```python
from build123d import *

# Parameters (mm, degrees)
SKETCH1_W               = 15
SKETCH1_H               = 32
SKETCH1_R               = 0.55
SKETCH1_W_2             = 12.4
SKETCH1_H_2             = 22.8
SERVO_MOUNT_PLATE_DEPTH = 4
SKETCH3_R               = 0.55
BOSS_EXTRUDE3_DEPTH     = 25
BOSS_EXTRUDE9_DEPTH     = 15
CUT_EXTRUDE3_START      = 1.5
CUT_EXTRUDE3_DEPTH      = 13.5
FILLET1_R               = 3
BODY_MOVE_COPY1_ANGLE   = 90


with BuildPart() as part:
    # Sketch1 → Servo Mount Plate (new body)
    with BuildSketch(Plane.XY):
        Rectangle(SKETCH1_W, SKETCH1_H)
        with Locations((0, 13.9)):
            Circle(SKETCH1_R, mode=Mode.SUBTRACT)
        with Locations((0, -13.9)):
            Circle(SKETCH1_R, mode=Mode.SUBTRACT)
        Rectangle(SKETCH1_W_2, SKETCH1_H_2, mode=Mode.SUBTRACT)
    extrude(amount=SERVO_MOUNT_PLATE_DEPTH)

    # Sketch3 → Boss-Extrude3 (add)
    # profile 1 of 2: a face of its own
    with BuildSketch(Plane.XY.offset(4)):
        Polygon((6.2, -11.4), (-6.2, -11.4), (-7.5, -11.4), (-7.5, -16), (7.5, -16), (7.5, -11.4), align=None)
        with Locations((0, -13.9)):
            Circle(SKETCH3_R, mode=Mode.SUBTRACT)
    # profile 2 of 2: a face of its own
    with BuildSketch(Plane.XY.offset(4)):
        with Locations((0, -13.9)):
            Circle(SKETCH3_R)
    extrude(amount=BOSS_EXTRUDE3_DEPTH)

    # Sketch5 → Boss-Extrude9 (add)
    with BuildSketch(Plane.XY.offset(14)):
        with BuildLine():
            Line((5.615385478, -4.685808185), (7.5, -6.00542948))
            Line((7.5, -6.00542948), (21.773725966, -16))
            Line((21.773725966, -16), (21.773725966, -5.013028701))
            Line((21.773725966, -5.013028701), (11.126345195, 2.442347577))
            ThreePointArc((11.126345195, 2.442347577), (9.098023831, -1.683915153), (5.615385478, -4.685808185))
        make_face()
        Polygon((21.773725966, -16), (7.5, -6.00542948), (7.5, -11.4), (7.5, -16), align=None)
        with BuildLine():
            Line((7.5, -11.4), (7.5, -6.00542948))
            Line((7.5, -6.00542948), (5.615385478, -4.685808185))
            ThreePointArc((5.615385478, -4.685808185), (0.865900109, -6.117354403), (-4.044697914, -5.415241232))
            Line((-4.044697914, -5.415241232), (-7.5, -11.4))
            Line((-7.5, -11.4), (7.5, -11.4))
        make_face()
    extrude(amount=BOSS_EXTRUDE9_DEPTH)

    # Sketch5<8> → Cut-Extrude3 (cut)
    with BuildSketch(Plane.XY.offset(14).offset(CUT_EXTRUDE3_START)):
        with BuildLine():
            Line((5.615385478, -4.685808185), (7.5, -6.00542948))
            Line((7.5, -6.00542948), (21.773725966, -16))
            Line((21.773725966, -16), (21.773725966, -5.013028701))
            Line((21.773725966, -5.013028701), (11.126345195, 2.442347577))
            ThreePointArc((11.126345195, 2.442347577), (9.098023831, -1.683915153), (5.615385478, -4.685808185))
        make_face()
    extrude(amount=CUT_EXTRUDE3_DEPTH, mode=Mode.SUBTRACT)

    # Fillet1
    fillet1_edges = [part.edges().sort_by_distance(p)[0] for p in [
        (6.85, -11.4, 4),
        (-6.85, -11.4, 4),
        (11.126345195, 2.442347577, 14.75),
        (21.773725966, -5.013028701, 14.75),
    ]]
    fillet(fillet1_edges, radius=FILLET1_R)


with BuildPart() as part_1:
    # Body-Move/Copy1: moved
    add(part.part.rotate(Axis((0, 0, 14.5), (1, 0, 0)), BODY_MOVE_COPY1_ANGLE))


solid = part_1.part
```
Verification items for the finished model (mm, model axes). A direction names the side the tool comes from. Give positions to 0.01 mm unless a question says otherwise; leave off trailing zeros. Order: outer loops, then holes, each group sorted by start corner. A loop starts at its lowest first (then second) coordinate and runs counter-clockwise, first axis right, second up. Notation, with made-up numbers: M 86.25,67.25 L 121.25,67.25 A15 ccw 121.25,94.25 Z; hole C 44,51.25 d8. An arc over 180 degrees is marked long. Return JSON: item names as keys, results as strings. Group by question number.
1) Section check A-A on z = 17. Record the cut outline in (x, y).
2) Mould release check, pull along X, two halves, no side actions. Record for faces 4 (the face through (-5.75, -6.9, 6.13)), 5 (the face through (0, 10.5, 0.6)), 6 (the face through (11.834, -0.261, 15.314)), 7 (the face through (6.84, 9.6, 3.96)): pulls with the +X half, pulls with the -X half, needs draft (parallel to the pull), parting line crosses it, or undercut.
3) Scan lines: line 1 (Z direction, x = 0, y = 13.1); line 2 (X direction, y = 12.5, z = 14.5); line 3 (X direction, y = 13.45, z = 28.4). Record each from-to range of solid material in increasing order.
4) Go/stop test with flat-tipped pins: pin 1 Ø4 at (x, y) = (15, -5.5) entering from +Z; pin 2 Ø12 at (x, y) = (6.5, -2) entering from +Z; pin 3 Ø7 at (y, z) = (10, 12.5) entering from +X. Record where each tip stops, or that it passes through.
5) Access from +Z, -Z, +X, -X, +Y, -Y to the whole of each face (thin tool, end or side, straight path). Record for faces 1 (the face through (-6.86, 9.6, 3.96)), 2 (the face through (15, -1, 9)), 3 (the face through (6.2, 13, 14)).
6) Section check B-B on x = -1.75. Record the cut outline in (y, z).
7) Section check D-D on y = 2.5. Record the cut outline in (x, z).
8) Section check C-C on z = 28.4. Record the cut outline in (x, y), and give its area (3 significant figures).
Answer block:
{
 "1": {"outline": "M -7.5,10.5 L -6.2,10.5 L -6.2,14.5 L -7.5,14.5 Z; M 6.2,10.5 L 7.5,10.5 L 7.5,14.5 L 6.2,14.5 Z"},
 "2": {"face 4": "pulls with the -X half", "face 5": "undercut", "face 6": "parting line crosses it", "face 7": "needs draft"},
 "3": {"line 1": "z = -1.5 to 0.05, 1.15 to 3.1, 25.9 to 27.85, 28.95 to 30.5", "line 2": "x = -7.5 to -6.2, 6.2 to 7.5", "line 3": "x = -7.5 to -0.55, 0.55 to 7.5"},
 "4": {"pin 1": "stops at z = 4.64", "pin 2": "stops at z = 15.37", "pin 3": "stops at x = 7.5"},
 "5": {"face 1": "+Z, +X, -X", "face 2": "+Z, +X, -Y", "face 3": "+Y"},
 "6": {"outline": "M -14.5,-1.5 L 14.5,-1.5 L 14.5,3.1 L 0.5,3.1 L 0.5,8.48 L -14.5,8.48 Z; M 10.5,25.9 L 14.5,25.9 L 14.5,30.5 L 10.5,30.5 Z"},
 "7": {"outline": "M -7.5,-1.5 L 7.5,-1.5 L 7.5,3.1 L -7.5,3.1 Z"},
 "8": {"outline": "M -7.5,10.5 L -0.55,10.5 L -0.55,14.5 L -7.5,14.5 Z; M 0.55,10.5 L 7.5,10.5 L 7.5,14.5 L 0.55,14.5 Z", "area": "55.6 mm^2"}
}
